The listing builds one solid part. Answer for the finished solid, in the listing's coordinates (mm). A direction names the side the tool comes from. Give positions to 0.01 mm unless a question says otherwise; leave off trailing zeros. Order: outer loops, then holes, each group sorted by start corner. A loop starts at its lowest first (then second) coordinate and runs counter-clockwise, first axis right, second up.
```python
from build123d import *

# Parameters (mm, degrees)
EXTRUDE_1_DEPTH     = 16
SKETCH_2_W          = 1.5
SKETCH_2_H          = 4.2
SKETCH_2_W_2        = 72.5
SKETCH_2_H_2        = 8.3
CUT_EXTRUDE_1_DEPTH = 109.463127375
FILLET_1_R          = 4.1


with BuildPart() as part:
    # 스케치1 → 보스-돌출1 (new body)
    with BuildSketch(Plane.XY):
        Polygon((-106, 0), (0, 0), (0, -16.5), (7.5, -16.5), (7.5, 5), (-106, 5), align=None)
    extrude(amount=EXTRUDE_1_DEPTH)

    # 스케치2 → 컷-돌출1 (cut, through all)
    with BuildSketch(Plane.XZ):
        with Locations((-101, 8)):
            Rectangle(SKETCH_2_W, SKETCH_2_H)
        with Locations((-47.25, 8)):
            Rectangle(SKETCH_2_W_2, SKETCH_2_H_2)
    extrude(amount=-CUT_EXTRUDE_1_DEPTH, mode=Mode.SUBTRACT)

    # 필렛1
    fillet_1_edges = [part.edges().sort_by_distance(p)[0] for p in [
        (-83.5, 2.5, 3.85),
        (-83.5, 2.5, 12.15),
        (-11, 2.5, 12.15),
        (-11, 2.5, 3.85),
    ]]
    fillet(fillet_1_edges, radius=FILLET_1_R)


solid = part.part
```
1) Straight lines are drawn through the part: probe 1 along X at (y, z) = (-4.25, 14); probe 2 along Y at (x, z) = (-10, 10); probe 3 along Z at (x, y) = (-70, 3.75). For each, find the intervals that lie inside material, in ascending order.
Geometry says:
probe 1: x = 0 to 7.5
probe 2: y = 0 to 5
probe 3: z = 0 to 3.85, 12.15 to 16
2) For a pull along X with two mould halves and no side action, classify faces 1 (the flat face through (-41, 1, 0)), 2 (the flat face through (7.5, -6, 8)), 3 (the cylindrical face through (-82.33, 2.54, 5.08)) as +X half, -X half, draft (parallel to the pull), parting line (faces both ways), or undercut.
Geometry says:
face 1: draft
face 2: +X half
face 3: undercut
3) Find section B-B (y = 1.5). Write down the section's boundary in (x, z), then the cut area to 3 significant figures.
Geometry says:
outline: (-106, 0) - (7.5, 0) - (7.5, 16) - (-106, 16) - close; hole (-101.75, 5.9) - (-100.25, 5.9) - (-100.25, 10.1) - (-101.75, 10.1) - close; hole (-83.5, 7.95) arc R4.1 ccw to (-79.4, 3.85) - (-15.1, 3.85) arc R4.1 ccw to (-11, 7.95) - (-11, 8.05) arc R4.1 ccw to (-15.1, 12.15) - (-79.4, 12.15) arc R4.1 ccw to (-83.5, 8.05) - close
area: 1,220 mm2
4) Find section C-C (z = 14). Write down the section's boundary in (x, y), then the cut area to 3 significant figures.
Geometry says:
outline: (-106, 0) - (0, 0) - (0, -16.5) - (7.5, -16.5) - (7.5, 5) - (-106, 5) - close
area: 691 mm2
5) Given P1, Ø2, axis at x = -30.5, z = 1.5, coming from the -Y side; P2, Ø8, axis at y = -10.5, z = 11.5, coming from the -X side, each flat-ended and moving along its own axis, determine where each tip first touches the part or whether it passes through.
Geometry says:
P1: stops at y = 0
P2: stops at x = 0
6) A tool of negligible diameter and unlimited length cuts with its end or side. For faces 4 (the flat face through (-41, 1, 16)), 5 (the flat face through (-48, 2, 12.15)), 6 (the flat face through (-54, 0, 13)), from which of +Z, -Z, +X, -X, +Y, -Y can it reach the whole face along a straight path? Write none if from no direction.
Geometry says:
face 4: +Z, +X, -X, +Y, -Y
face 5: +Y, -Y
face 6: +Z, -Z, -X, -Y
7) Find section A-A (x = -51). Write down the section's boundary in (y, z).
Geometry says:
outline: (0, 0) - (5, 0) - (5, 3.85) - (0, 3.85) - close; (0, 12.15) - (5, 12.15) - (5, 16) - (0, 16) - close
8) Find section D-D (x = -5). Write down the section's boundary in (y, z).
Geometry says:
outline: (0, 0) - (5, 0) - (5, 16) - (0, 16) - close
